from build123d import *

# Parameters (mm, degrees)
F1_DEPTH = 1000
F3_DEPTH = 65.001
F5_DEPTH = 125.001
F6_R     = 9
F7_DEPTH = 7.5
F8_R     = 9
F9_DEPTH = 7.5


with BuildPart() as f1:
    # F0 (on Front) → F1 (new body)
    with BuildSketch(Plane.XZ):
        with BuildLine():
            Line((-25.16784, 62.5), (-25.16784, -62.5))
            Line((-25.16784, -62.5), (39.83216, -62.5))
            Line((39.83216, -62.5), (39.83216, -55))
            Line((39.83216, -55), (-12.46784, -55))
            ThreePointArc((-12.46784, -55), (-18.124695, -52.656854), (-20.46784, -47))
            Line((-20.46784, -47), (-20.46784, 47))
            ThreePointArc((-20.46784, 47), (-18.124695, 52.656854), (-12.46784, 55))
            Line((-12.46784, 55), (39.83216, 55))
            Line((39.83216, 55), (39.83216, 62.5))
            Line((39.83216, 62.5), (-25.16784, 62.5))
        make_face()
    extrude(amount=F1_DEPTH)

    # F2 (on face) → F3 (cut, through all)
    with BuildSketch(Plane(origin=(-25.16784, 0, 0), x_dir=(0, -1, 0), z_dir=(-1, 0, 0))):
        Polygon((125, 62.5), (0, 62.5), (0, -62.5), align=None)
    extrude(amount=-F3_DEPTH, mode=Mode.SUBTRACT)

    # F4 (on face) → F5 (cut, through all)
    with BuildSketch(Plane.XY.offset(62.5)):
        Polygon((-25.16784, -1000), (39.83216, -1000), (39.83216, -935), align=None)
    extrude(amount=-F5_DEPTH, mode=Mode.SUBTRACT)

    # F6 (on face) → F7 (cut, through all)
    with BuildSketch(Plane.XY.offset(62.5)):
        with Locations((7.33216, -548)):
            Circle(F6_R)
        with Locations((7.33216, -650)):
            Circle(F6_R)
    extrude(amount=-F7_DEPTH, mode=Mode.SUBTRACT)

    # F8 (on face) → F9 (cut, through all)
    with BuildSketch(Plane.XY.offset(62.5)):
        with Locations((7.33216, -300)):
            Circle(F8_R)
        with Locations((7.33216, -402)):
            Circle(F8_R)
    extrude(amount=-F9_DEPTH, mode=Mode.SUBTRACT)


solid = f1.part
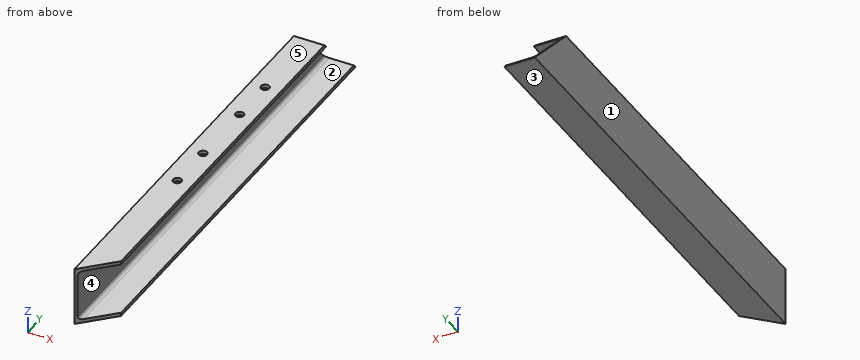
For this review, take the finished solid that the model builds, in its own axes (mm). Face numbers are marked on the shaded views. A direction names the side the tool comes from. Round coordinates to 2 decimals unless told otherwise and drop trailing zeros. Loops run counter-clockwise (first coordinate to the right, second up) from the corner with the lowest first, then second, coordinate; pieces in that order, holes last. Notation, with made-up numbers: (-16.75, 23.5) - (10.25, 23.5) arc R3 ccw to (10.25, 27.5) - close; hole circle Ø7 at (44, 26). An arc over 180 degrees is marked (long way). One line per item, written item: value. Start each with the question number.
Item 1: For the marked faces 1 and 2, list the 3-axis set-ups (+Z, -Z, +X, -X, +Y, -Y) from which the entire face can be reached by the end or side of a thin tool; tool diameter is ignored.
Item 2: Clearance check with flat-ended pins moving along their axes: pin 1 Ø12 at (x, y) = (-8, -103.5) entering from +Z; pin 2 Ø10 at (x, z) = (-18.5, 12.5) entering from +Y; pin 3 Ø8 at (y, z) = (-306, -34) entering from +X. State where each tip first meets the part, or that it passes through.
Item 3: Take a section at D-D (z = 19.5). Give the boundary of the cut face in (x, y).
Item 4: Take a section at B-B (z = -34). Give the boundary of the cut face in (x, y).
Item 5: Take a section at C-C (y = -206). Give the boundary of the cut face in (x, z), plus the area to 3 significant figures.
Item 6: Take a section at A-A (y = -650). Give the boundary of the cut face in (x, z), plus the area to 3 significant figures.
Item 7: The part is to be moulded in two halves that separate along Z. For the marked faces 3, 4 and 5, say which applies: +Z half, -Z half, draft (parallel to the pull), parting line (faces both ways), or undercut.
Item 8: For L1, parallel to Z at x = 28, y = -316.5; L2, parallel to X at y = -548, z = 58.25; L3, parallel to X at y = -142, z = -19.5, list the stretches that pass through material, from the lowest coordinate up.
Answer below:
1. face 1: +Z, -Z, -X, +Y, -Y
1. face 2: +X, +Y, -Y
2. pin 1: stops at z = -54.85
2. pin 2: stops at y = -70.4
2. pin 3: stops at x = -20.47
3. outline: (-25.17, -1000) - (-20.47, -995.3) - (-20.47, -82) - (-25.17, -82) - close
4. outline: (-25.17, -1000) - (-20.47, -995.3) - (-20.47, -28.5) - (-25.17, -28.5) - close
5. outline: (-25.17, -62.5) - (39.83, -62.5) - (39.83, -55) - (-12.47, -55) arc R8 cw to (-20.47, -47) - (-20.47, 47) arc R8 cw to (-12.47, 55) - (39.83, 55) - (39.83, 62.5) - (-25.17, 62.5) - close
5. area: 1,520 mm2
6. outline: (-25.17, -62.5) - (39.83, -62.5) - (39.83, -55) - (-12.47, -55) arc R8 cw to (-20.47, -47) - (-20.47, 47) arc R8 cw to (-12.47, 55) - (-1.67, 55) - (-1.67, 62.5) - (-25.17, 62.5) - close; (16.33, 55) - (39.83, 55) - (39.83, 62.5) - (16.33, 62.5) - close
6. area: 1,380 mm2
7. face 3: -Z half
7. face 4: undercut
7. face 5: +Z half
8. L1: z = -62.5 to -55, 55 to 62.5
8. L2: x = -25.17 to -1.67, 16.33 to 39.83
8. L3: x = -25.17 to -20.47
